```python
from build123d import *

# Parameters (mm, degrees)
EXTRUDE_2_DEPTH                = 5
SKETCH_4_W                     = 8.676470589
SKETCH_4_H                     = 35
SKETCH_4_W_2                   = 8.676470588
EXTRUDE_15_DEPTH               = 35
CUT_EXTRUDE_1_DEPTH            = 45
SKETCH_6_R                     = 15
CUT_EXTRUDE_2_DEPTH            = 45
FILLET_1_R                     = 5
EXTRUDE_START                  = -1
SKETCH_7_R                     = 15
SKETCH_7_R_2                   = 13
EXTRUDE_16_DEPTH               = 1
SKETCH_8_R                     = 15
SKETCH_8_R_2                   = 13
EXTRUDE_17_DEPTH               = 1
SPLIT_BODIES_1_SURFACE_1_BACK  = 86
SPLIT_BODIES_1_SURFACE_1_DEPTH = 172
SPLIT_BODIES_1_SURFACE_2_BACK  = 86
SPLIT_BODIES_1_SURFACE_2_DEPTH = 172
HOLE_WIZARD_1_D                = 5.3
HOLE_WIZARD_1_CBORE_D          = 10.5
HOLE_WIZARD_1_CBORE_DEPTH      = 3


with BuildPart() as part:
    # 草图2 → 凸台-拉伸2 (new body)
    with BuildSketch(Plane.XY):
        Polygon((7.726423565, 24.338235294), (-14.773576435, 24.338235294), (-14.773576435, -35.661764706), (7.726423565, -35.661764706), (7.726423565, -23.161764706), (-6.097105846, -23.161764706), (-6.097105846, 11.838235294), (7.726423565, 11.838235294), align=None)
        Polygon((30.226423565, 24.338235294), (7.726423565, 24.338235294), (7.726423565, 11.838235294), (21.549952977, 11.838235294), (21.549952977, -23.161764706), (7.726423565, -23.161764706), (7.726423565, -35.661764706), (30.226423565, -35.661764706), align=None)
    extrude(amount=EXTRUDE_2_DEPTH)

    # 草图4 → 凸台-拉伸15 (add)
    with BuildSketch(Plane.XY.offset(5)):
        with Locations((-10.435341141, -5.661764706)):
            Rectangle(SKETCH_4_W, SKETCH_4_H)
        with Locations((25.888188271, -5.661764706)):
            Rectangle(SKETCH_4_W_2, SKETCH_4_H)
    extrude(amount=EXTRUDE_15_DEPTH)

    # 草图5 → 切除-拉伸1 (cut)
    with BuildSketch(Plane.ZY.offset(14.773576435)):
        with BuildLine():
            Line((40, -23.161764706), (40, -5.661764706))
            ThreePointArc((40, -5.661764706), (34.874368671, -18.036133377), (22.5, -23.161764706))
            Line((22.5, -23.161764706), (40, -23.161764706))
        make_face()
        with BuildLine():
            ThreePointArc((22.5, 11.838235294), (34.874368671, 6.712603965), (40, -5.661764706))
            Line((40, -5.661764706), (40, 11.838235294))
            Line((40, 11.838235294), (22.5, 11.838235294))
        make_face()
    extrude(amount=-CUT_EXTRUDE_1_DEPTH, mode=Mode.SUBTRACT)

    # 草图6 → 切除-拉伸2 (cut)
    with BuildSketch(Plane.ZY.offset(14.773576435)):
        with Locations((22.5, -5.661764706)):
            Circle(SKETCH_6_R)
    extrude(amount=-CUT_EXTRUDE_2_DEPTH, mode=Mode.SUBTRACT)

    # 圆角1
    fillet_1_edges = [part.edges().sort_by_distance(p)[0] for p in [
        (-6.097105846, 11.838235294, 2.5),
        (-6.097105846, -23.161764706, 2.5),
        (21.549952977, -23.161764706, 2.5),
        (21.549952977, 11.838235294, 2.5),
    ]]
    fillet(fillet_1_edges, radius=FILLET_1_R)

    # 草图7 → 凸台-拉伸16 (add)
    with BuildSketch(Plane(origin=(-6.097105846, 0, 0), x_dir=(0, 0, -1), z_dir=(1, 0, 0)).offset(EXTRUDE_START)):
        with Locations(Location((-22.5, -5.661764706, 0), (0, 0, 180))):
            Circle(SKETCH_7_R)
        with Locations((-22.5, -5.661764706)):
            Circle(SKETCH_7_R_2, mode=Mode.SUBTRACT)
    extrude(amount=EXTRUDE_16_DEPTH)

    # 草图8 → 凸台-拉伸17 (add)
    with BuildSketch(Plane.ZY.offset(-21.549952977)):
        with Locations((22.5, -5.661764706)):
            Circle(SKETCH_8_R)
        with Locations(Location((22.5, -5.661764706, 0), (0, 0, 180))):
            Circle(SKETCH_8_R_2, mode=Mode.SUBTRACT)
    extrude(amount=-EXTRUDE_17_DEPTH)


with BuildPart() as body_2:
    # Split Bodies 1: the piece behind the surface
    add(part.part)
    # Split Bodies 1 surface: a surface, the sketch's curves swept straight by 172 mm
    with BuildLine(Plane.XY.offset(5).offset(-SPLIT_BODIES_1_SURFACE_1_BACK), mode=Mode.PRIVATE) as split_bodies_1_surface_1_path:
        Line((7.726423565, 24.338235294), (7.726423565, -35.661764706))
    split_bodies_1_surface_1 = Shell.extrude(split_bodies_1_surface_1_path.wire(), (0 * SPLIT_BODIES_1_SURFACE_1_DEPTH, 0 * SPLIT_BODIES_1_SURFACE_1_DEPTH, 1 * SPLIT_BODIES_1_SURFACE_1_DEPTH))
    split(bisect_by=split_bodies_1_surface_1, keep=Keep.BOTTOM)


with BuildPart() as part_1:
    add(part.part)

    # Split Bodies 1: split by a surface, the side it looks to stays
    # Split Bodies 1 surface: a surface, the sketch's curves swept straight by 172 mm
    with BuildLine(Plane.XY.offset(5).offset(-SPLIT_BODIES_1_SURFACE_2_BACK), mode=Mode.PRIVATE) as split_bodies_1_surface_2_path:
        Line((7.726423565, 24.338235294), (7.726423565, -35.661764706))
    split_bodies_1_surface_2 = Shell.extrude(split_bodies_1_surface_2_path.wire(), (0 * SPLIT_BODIES_1_SURFACE_2_DEPTH, 0 * SPLIT_BODIES_1_SURFACE_2_DEPTH, 1 * SPLIT_BODIES_1_SURFACE_2_DEPTH))
    split(bisect_by=split_bodies_1_surface_2, keep=Keep.TOP)

    # 大小平盘开槽螺钉柱孔1 (through all)
    with Locations(Plane(origin=(20.226423565, -29.411764706, 5), x_dir=(1, 0, 0), z_dir=(0, 0, 1))):
        with Locations((0, 0), (0, 47.5)):
            CounterBoreHole(HOLE_WIZARD_1_D / 2, HOLE_WIZARD_1_CBORE_D / 2, HOLE_WIZARD_1_CBORE_DEPTH)


solid = part_1.part
```
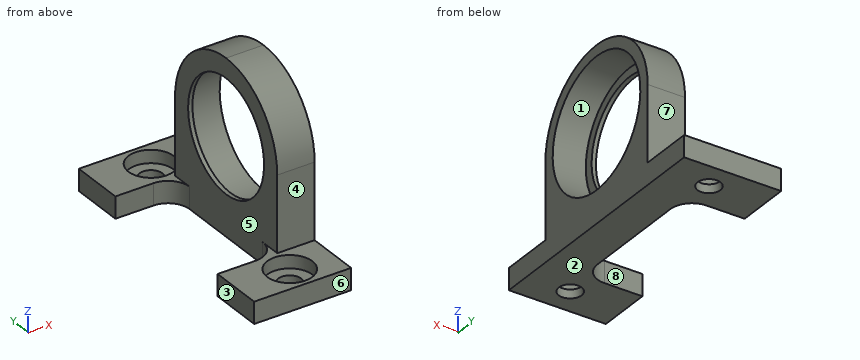
Geometry: final body of the model. Coordinates: model frame, mm. Face numbers are marked on the shaded views. A direction names the side the tool comes from. Round coordinates to 2 decimals unless told otherwise and drop trailing zeros. Order: outer loops, then holes, each group sorted by start corner. A loop starts at its lowest first (then second) coordinate and runs counter-clockwise, first axis right, second up. Notation, with made-up numbers: (20.25, -3) - (31.25, -3) arc R16 ccw to (31.25, 10) - close; hole circle Ø2 at (73.25, 29.25). An arc over 180 degrees is marked (long way). Use CSV: the item, a comma, the result in double quotes. Start each with the question number.
Q1. Mould query, pull axis Z, two halves, no side actions, for the marked faces 1, 2 and 3. Classes: +Z half, -Z half, draft (parallel to the pull), parting line (faces both ways), or undercut.
Q2. First-contact query: pin 1 (2.5 mm diameter, centred on x = 25.5, z = 9.5, fed in from -Y); pin 2 (9 mm diameter, centred on x = 15, y = -30.5, fed in from +Z); pin 3 (4.5 mm diameter, centred on x = 24, z = 13.5, fed in from +Y). Flat tips, straight axial feed; report the tip coordinate or a pass-through.
Q3. Access query for the marked faces 4, 5, 6, 7 and 8. Directions: +Z, -Z, +X, -X, +Y, -Y. A direction counts if a zero-diameter tool reaches every point of the face in a straight line with its end or side. Return the directions, or none.
Q4. Section query D-D (x = 27.25). Return loops of the section in (y, z), and give its area (3 significant figures).
Q5. Section query B-B (z = 4). Return loops of the section in (x, y), and give its area (3 significant figures).
Q6. Material intervals for line 1 along Y through (x, z) = (28.75, 22.5); line 2 along Y through (x, z) = (28, 29); line 3 along Z through (x, y) = (19.75, 14), sorted ascending. Write a range as from..to.
Q7. Section query C-C (x = 20.5). Return loops of the section in (y, z).
Q8. Section query A-A (x = 12.5). Return loops of the section in (y, z).
Result set:
1,face 1,"undercut"
1,face 2,"-Z half"
1,face 3,"draft"
2,pin 1,"stops at y = -23.16"
2,pin 2,"stops at z = 5"
2,pin 3,"stops at y = 11.84"
3,face 4,"+Z, +X, -X, -Y"
3,face 5,"+Z, -X"
3,face 6,"+Z, -Z, +X, -X, -Y"
3,face 7,"+Z, +X, -X, +Y"
3,face 8,"+Z, -Z, -X"
4,outline,"(-35.66, 0) - (24.34, 0) - (24.34, 5) - (11.84, 5) - (11.84, 22.5) arc R17.5 ccw to (-23.16, 22.5) - (-23.16, 5) - (-35.66, 5) - close; hole circle Ø30 at (-5.66, 22.5)"
4,area,"687 mm2"
5,outline,"(7.73, -35.66) - (30.23, -35.66) - (30.23, 24.34) - (7.73, 24.34) - (7.73, 11.84) - (16.55, 11.84) arc R5 cw to (21.55, 6.84) - (21.55, -18.16) arc R5 cw to (16.55, -23.16) - (7.73, -23.16) - close; hole circle Ø10.5 at (20.23, -29.41); hole circle Ø10.5 at (20.23, 18.09)"
5,area,"704 mm2"
6,line 1,"y = -23.16..-20.66, 9.34..11.84"
6,line 2,"y = -21.91..-19.18, 7.86..10.59"
6,line 3,"z = 0..2"
7,outline,"(-35.66, 0) - (-32.05, 0) - (-32.05, 2) - (-34.65, 2) - (-34.65, 5) - (-35.66, 5) - close; (-26.78, 0) - (-21.23, 0) - (-21.23, 5) - (-24.17, 5) - (-24.17, 2) - (-26.78, 2) - close; (9.9, 0) - (15.45, 0) - (15.45, 2) - (12.85, 2) - (12.85, 5) - (9.9, 5) - close; (20.72, 0) - (24.34, 0) - (24.34, 5) - (23.33, 5) - (23.33, 2) - (20.72, 2) - close"
8,outline,"(-35.66, 0) - (-23.16, 0) - (-23.16, 5) - (-35.66, 5) - close; (11.84, 0) - (24.34, 0) - (24.34, 5) - (11.84, 5) - close"
